Autodesk Inventor part; units mm, degrees
ref_plane "YZ Plane" through (0, 0, 0) normal (1, 0, 0) x (0, 1, 0)
ref_plane "XZ Plane" through (0, 0, 0) normal (0, 1, 0) x (-1, 0, 0)
ref_plane "XY Plane" through (0, 0, 0) normal (0, 0, 1) x (1, 0, 0)
sketch "Esquisse1" plane through (0, 0, 0) normal (0, 0, 1) x (1, 0, 0)
  line L0 (0, 0) -> (19, 0)
  line L1 (19, 0) -> (19, 27)
  line L2 (19, 27) -> (0, 27)
  line L3 (0, 27) -> (0, 0)
  dimension "d0" = 27
  dimension "d1" = 19
extrude "Extrusion1" add sketch "Esquisse1" along normal blind 26
sketch "Esquisse2" plane through (0, 27, 0) normal (0, 1, 0) x (1, 0, 0)
  line L0 (19, 0) -> (2, 0)
  line L1 (2, 0) -> (2, -14)
  line L2 (2, -14) -> (19, -14)
  line L3 (19, -14) -> (19, 0)
  line L4 (0, 0) -> (0, -26)
  line L5 (19, 0) -> (19, -26)
  line L6 (0, -26) -> (19, -26)
  line L7 (19, -26) -> (19, -16)
  line L8 (19, -16) -> (0, -16)
  line L9 (0, -16) -> (0, -26)
  dimension "d4" = 2
  dimension "d5" = 2
  dimension "d6" = 14
  dimension "d7" = 10
extrude "Extrusion2" cut sketch "Esquisse2" against normal blind 22
sketch "Esquisse3" plane through (0, 5, 0) normal (0, 1, 0) x (1, 0, 0)
  circle A0 centre (3.75, -21) radius 1.5
  circle A1 centre (15.25, -21) radius 1.5
  line L0 (0, -16) -> (19, -16)
  line L1 (19, -16) -> (19, -26)
  line L2 (0, -26) -> (0, -16)
  point P0 (0, 0)
  dimension "d10" = 3
  dimension "d11" = 5
  dimension "d12" = 11.5
  dimension "d13" = 19
  dimension "d14" = 3.75
extrude "Extrusion3" cut sketch "Esquisse3" against normal through all
sketch "Esquisse4" plane through (0, 5, 0) normal (0, 1, 0) x (1, 0, 0)
  circle A0 centre (3.75, -21) radius 1.5
  line L0 (3.75, -16.9585) -> (7.25, -18.9793)
  line L1 (7.25, -18.9793) -> (7.25, -23.0207)
  line L2 (7.25, -23.0207) -> (3.75, -25.0415)
  line L3 (3.75, -25.0415) -> (0.25, -23.0207)
  line L4 (0.25, -23.0207) -> (0.25, -18.9793)
  line L5 (0.25, -18.9793) -> (3.75, -16.9585)
  circle A1 centre (15.25, -21) radius 1.5
  line L6 (15.25, -16.9585) -> (18.75, -18.9793)
  line L7 (18.75, -18.9793) -> (18.75, -23.0207)
  line L8 (18.75, -23.0207) -> (15.25, -25.0415)
  line L9 (15.25, -25.0415) -> (11.75, -23.0207)
  line L10 (11.75, -23.0207) -> (11.75, -18.9793)
  line L11 (11.75, -18.9793) -> (15.25, -16.9585)
  point P0 (0, 0)
  dimension "d17" = 7
extrude "Extrusion4" cut sketch "Esquisse4" against normal blind 2.5
fillet "Congé1" radius 5 2 edges at (1, 27, 0) (19, 27, 15)
equation "\"d14\" = -0.5 * d12 + 0.5 * d13"
properties part number "EquerreBatterieGauche" material "Plastique ABS"
Can you work these out from the model? Positions are in its coordinate system, mm. A direction names the side the tool comes from. Give positions to 0.01 mm unless a question says otherwise; leave off trailing zeros. Loops run counter-clockwise (first coordinate to the right, second up) from the corner with the lowest first, then second, coordinate; pieces in that order, holes last. Notation, with made-up numbers: M -13,15 L 3,15 A23 ccw 3,52 Z; hole C 55.25,18.5 d9. An arc over 180 degrees is marked long. One line per item, written item: value. Start each with the question number.
1) If we section it at C-C, the plane x = 14.75: Write out the boundary of the cut face in (y, z).
2) If I drill on line 1 (X direction, y = 0.95, z = 21); line 2 (Z direction, x = 3.75, y = 1.95); line 3 (Y direction, x = 9.5, z = 8.75), over which ranges is the centre line in solid material (lowest first)? Write a range as [from, to].
3) If we section it at D-D, the plane y = 11.25: Write out the boundary of the cut face in (x, z).
4) If we section it at A-A, the plane z = 21: Write out the boundary of the cut face in (x, y).
5) If we section it at B-B, the plane x = 8.75: Write out the boundary of the cut face in (y, z).
6) I'm going to push flat-ended pins straight in: pin 1 (7 mm diameter, centred on x = 7, z = 3.5, fed in from +Y); pin 2 (1 mm diameter, centred on x = 4, y = 18.5, fed in from +Z); pin 3 (5 mm diameter, centred on x = 10.5, y = 19, fed in from -Z); pin 4 (1.8 mm diameter, centred on x = 3.75, z = 21, fed in from -Y). Where does each tip first touch, or does it pass through?
7) On a 3-axis mill with a long thin cutter (end or side, diameter ignored), from which of +Z, -Z, +X, -X, +Y, -Y can I reach the whole of each face in a straight line? I mean faces 1 (the face through (10, 5, 7)), 2 (the face through (5.476, 3.768, 17.955)), 3 (the face through (9, 5, 21)). Say none if no direction works.
8) Thinking about a two-plate mould opening in X: for faces 4 (the face through (0, 14, 10)), 5 (the face through (9, 0, 13)), 6 (the face through (1.98, 3.77, 17.98)), 7 (the face through (2.024, 3.768, 24.045)), which applies, +X half, -X half, draft (parallel to the pull), parting line (faces both ways), or undercut?
Completed:
1. outline: M 0,0 L 5,0 L 5,14 L 26.94,14 L 26.94,16 L 5,16 L 5,17.25 L 2.5,17.25 L 2.5,19.59 L 0,19.59 Z; M 0,22.41 L 2.5,22.41 L 2.5,24.75 L 5,24.75 L 5,26 L 0,26 Z
2. line 1: x = [0, 2.25], [5.25, 13.75], [16.75, 19]
2. line 2: z = [0, 19.5], [22.5, 26]
2. line 3: y = [0, 5]
3. outline: M 0,0 L 2,0 L 2,14 L 19,14 L 19,16 L 0,16 Z
4. outline: M 0,0 L 2.25,0 L 2.25,2.5 L 0.25,2.5 L 0.25,5 L 0,5 Z; M 5.25,0 L 13.75,0 L 13.75,2.5 L 11.75,2.5 L 11.75,5 L 7.25,5 L 7.25,2.5 L 5.25,2.5 Z; M 16.75,0 L 19,0 L 19,5 L 18.75,5 L 18.75,2.5 L 16.75,2.5 Z
5. outline: M 0,0 L 5,0 L 5,14 L 27,14 L 27,16 L 5,16 L 5,26 L 0,26 Z
6. pin 1: stops at y = 5
6. pin 2: stops at z = 16
6. pin 3: stops at z = 14
6. pin 4: passes through
7. face 1: -Z, +X, +Y
7. face 2: +Y
7. face 3: +Z, +X, -X, +Y
8. face 4: -X half
8. face 5: draft
8. face 6: undercut
8. face 7: undercut
